Here's how the part is built. I have some questions about the finished solid (model axes, mm). Face numbers are marked on the shaded views. A direction names the side the tool comes from. Coordinates: 2 decimals unless noted, no trailing zeros. Write each loop counter-clockwise with the first axis right and the second up, starting at its lowest first coordinate (ties: lowest second). Pieces come first, ordered by that corner, then holes.
(1) Which directions (+Z, -Z, +X, -X, +Y, -Y) give clear straight access to the entire face, cutting with the end or side of a thin tool? Please do the marked faces 1, 2 and 3.
(2) For pin 1 Ø3 at (x, z) = (-12.5, 8) entering from +Y; pin 2 Ø4 at (y, z) = (-6.5, 16) entering from -X; pin 3 Ø2 at (x, y) = (-15.5, -8) entering from -Z, each with a flat end and sliding along its axis, tell me the tip position at first contact or that it passes through.
(3) Please list where these lines run through material, in increasing order: probe 1 along Z at (x, y) = (-7.5, -17); probe 2 along Z at (x, y) = (-19.5, -13.5); probe 3 along Y at (x, z) = (-9.25, 19.25).
(4) Imagine slicing it at D-D, the plane z = 4.5. List the corners of the cut face in (x, y) for me.
(5) Imagine slicing it at A-A, the plane y = -8. List the corners of the cut face in (x, z) for me, plus the area to 3 significant figures.
(6) Imagine slicing it at C-C, the plane z = 23.25. List the corners of the cut face in (x, y) for me, plus the area to 3 significant figures.
(7) Imagine slicing it at B-B, the plane x = -2.75. List the corners of the cut face in (y, z) for me.
```python
from build123d import *

# Parameters (mm, degrees)
BOSS_EXTRUDE1_DEPTH = 10
BOSS_EXTRUDE2_DEPTH = 15


with BuildPart() as part:
    # Sketch1 → Boss-Extrude1 (new body)
    with BuildSketch(Plane.XY):
        with BuildLine():
            Line((-30, -25), (0, 0))
            Line((0, 0), (0, -15))
            ThreePointArc((0, -15), (-2.928932188, -22.071067812), (-10, -25))
            Line((-10, -25), (-30, -25))
        make_face()
    extrude(amount=BOSS_EXTRUDE1_DEPTH)

    # Sketch3 → Boss-Extrude2 (add)
    with BuildSketch(Plane.XY.offset(10)):
        with BuildLine():
            ThreePointArc((-30, -25), (-19.624638361, -6.950433967), (0, 0))
            ThreePointArc((0, 0), (-10.375361639, -18.049566033), (-30, -25))
        make_face()
    extrude(amount=BOSS_EXTRUDE2_DEPTH)


solid = part.part
```
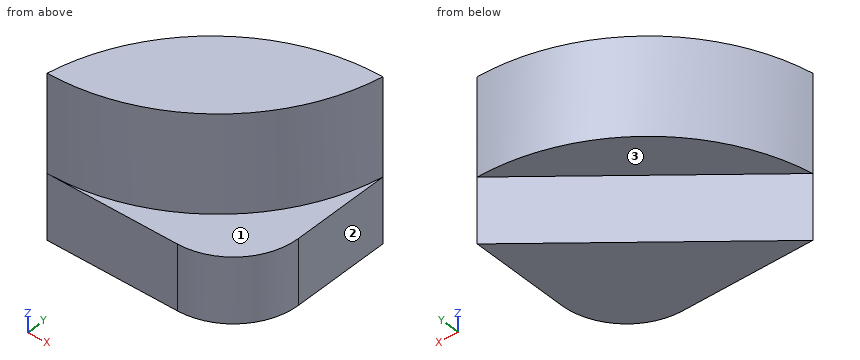
Recorded:
1. face 1: +Z, +X, -Y
1. face 2: +Z, -Z, +X, +Y, -Y
1. face 3: -Z, -X, +Y
2. pin 1: stops at y = -9.17
2. pin 2: stops at x = -21.34
2. pin 3: stops at z = 10
3. probe 1: z = 0 to 10
3. probe 2: z = 10 to 25
3. probe 3: y = -17.06 to -1.33
4. outline: (-30, -25) - (-10, -25) arc R10 ccw to (0, -15) - (0, 0) - close
5. outline: (-20.82, 10) - (-9.6, 10) - (-9.6, 0) - (0, 0) - (0, 10) - (-2.54, 10) - (-2.54, 25) - (-20.82, 25) - close
5. area: 370 mm2
6. outline: (-30, -25) arc R30 ccw to (0, 0) arc R30 ccw to start
6. area: 386 mm2
7. outline: (-21.89, 0) - (-2.29, 0) - (-2.29, 10) - (-0.09, 10) - (-0.09, 25) - (-8.42, 25) - (-8.42, 10) - (-21.89, 10) - close
